For this review, take the finished solid that the model builds, in its own axes (mm). Face numbers are marked on the shaded views. A direction names the side the tool comes from. Round coordinates to 2 decimals unless told otherwise and drop trailing zeros. Write each loop counter-clockwise with the first axis right and the second up, starting at its lowest first coordinate (ties: lowest second). Pieces come first, ordered by that corner, then holes. Notation, with made-up numbers: (63, 82.5) - (98, 82.5) arc R18 cw to (98, 106.5) - close; hole circle Ø6 at (-36, -12.5). An arc over 180 degrees is marked (long way). Answer in a Markdown table with one row per item. Add a question column.
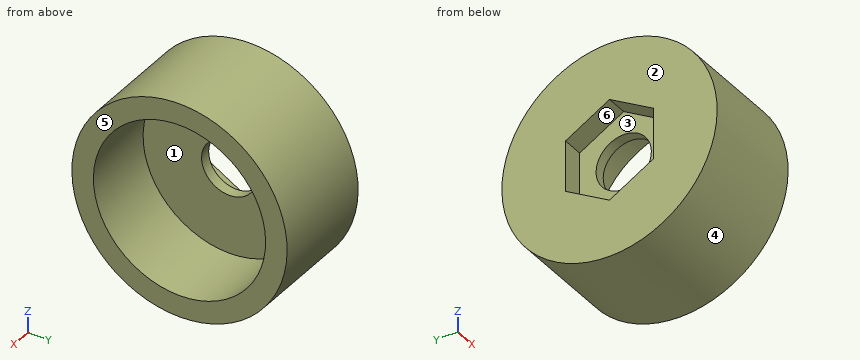
from build123d import *

# Parameters (mm, degrees)
ESBO_O1_R                = 50
RESSALTO_EXTRUS_O1_DEPTH = 50
ESBO_O2_R                = 40
CORTE_EXTRUS_O1_DEPTH    = 35
CORTE_EXTRUS_O2_DEPTH    = 10
ESBO_O4_R                = 12.832707742
CORTE_EXTRUS_O3_DEPTH    = 82.240384046


with BuildPart() as part:
    # Esboço1 → Ressalto-extrusão1 (new body)
    with BuildSketch(Plane(origin=(0, 0, 0), x_dir=(0, 0, -1), z_dir=(1, 0, 0))):
        Circle(ESBO_O1_R)
    extrude(amount=RESSALTO_EXTRUS_O1_DEPTH)

    # Esboço2 → Corte-extrusão1 (cut)
    with BuildSketch(Plane(origin=(50, 0, 0), x_dir=(0, 0, -1), z_dir=(1, 0, 0))):
        Circle(ESBO_O2_R)
    extrude(amount=-CORTE_EXTRUS_O1_DEPTH, mode=Mode.SUBTRACT)

    # Esboço3 → Corte-extrusão2 (cut)
    with BuildSketch(Plane.ZY):
        Polygon((-11.812450534, 20.459764487), (11.812450534, 20.459764487), (23.624901068, 0), (11.812450534, -20.459764487), (-11.812450534, -20.459764487), (-23.624901068, 0), align=None)
    extrude(amount=-CORTE_EXTRUS_O2_DEPTH, mode=Mode.SUBTRACT)

    # Esboço4 → Corte-extrusão3 (cut, through all)
    with BuildSketch(Plane.ZY.offset(-10)):
        Circle(ESBO_O4_R)
    extrude(amount=-CORTE_EXTRUS_O3_DEPTH, mode=Mode.SUBTRACT)


solid = part.part
Q1. To check wall thickness, follow probe 1 along Y at (x, z) = (12.85, 0); probe 2 along Y at (x, z) = (24, 0); probe 3 along X at (y, z) = (3.5, -29). State the ranges of each line that lie inside material, in increasing order.
Q2. Add section C-C on y = -36. State the section outline as (x, z) points.
Q3. Draft analysis for pull direction Y (two halves, no side actions). For the marked faces 4, 5 and 6, state which applies: released by +Y, released by -Y, zero draft, split by the parting line, or undercut.
Q4. Insertion check: pin 1 Ø6 at (x, y) = (32.5, 19) entering from +Z; pin 2 Ø8 at (x, z) = (5, 4) entering from -Y; pin 3 Ø8 at (x, y) = (40, 15) entering from +Z (3 decimals); pin 4 Ø1.5 at (y, z) = (-8.5, -19) entering from -X. Each pin has a flat end and moves straight along its axis. Give the tip position at first contact, or say it passes through.
Q5. Tool access review of the marked faces 1, 2 and 3: name each direction out of +Z, -Z, +X, -X, +Y, -Y from which nothing blocks a thin tool from reaching the whole face with its end or side.
Q6. Add section D-D on z = 19.5. State the section outline as (x, y) points.
Q7. Add section A-A on z = 0. State the section outline as (x, y) points, then the cut area to 3 significant figures.
Q8. Add section B-B on x = 4. State the section outline as (y, z) points, then the cut area to 3 significant figures.
Answer sheet:
| question | item | result |
|---|---|---|
| 1 | probe 1 | y = -50 to -12.83, 12.83 to 50 |
| 1 | probe 2 | y = -50 to -40, 40 to 50 |
| 1 | probe 3 | x = 0 to 15 |
| 2 | outline | (0, -34.7) - (50, -34.7) - (50, -17.44) - (15, -17.44) - (15, 17.44) - (50, 17.44) - (50, 34.7) - (0, 34.7) - close |
| 3 | face 4 | split by the parting line |
| 3 | face 5 | zero draft |
| 3 | face 6 | undercut |
| 4 | pin 1 | stops at z = 47.37 |
| 4 | pin 2 | stops at y = -50 |
| 4 | pin 3 | stops at z = 48.775 |
| 4 | pin 4 | stops at x = 0 |
| 5 | face 1 | +X |
| 5 | face 2 | +Z, -Z, -X, +Y, -Y |
| 5 | face 3 | -X |
| 6 | outline | (0, -46.04) - (50, -46.04) - (50, -34.92) - (15, -34.92) - (15, 34.92) - (50, 34.92) - (50, 46.04) - (0, 46.04) - (0, 7.14) - (10, 7.14) - (10, -7.14) - (0, -7.14) - close |
| 7 | outline | (0, -50) - (50, -50) - (50, -40) - (15, -40) - (15, -12.83) - (10, -12.83) - (10, -20.46) - (0, -20.46) - close; (0, 20.46) - (10, 20.46) - (10, 12.83) - (15, 12.83) - (15, 40) - (50, 40) - (50, 50) - (0, 50) - close |
| 7 | area | 1,660 mm² |
| 8 | outline | circle Ø100 at (0, 0); hole (-20.46, -11.81) - (0, -23.62) - (20.46, -11.81) - (20.46, 11.81) - (0, 23.62) - (-20.46, 11.81) - close |
| 8 | area | 6,400 mm² |
